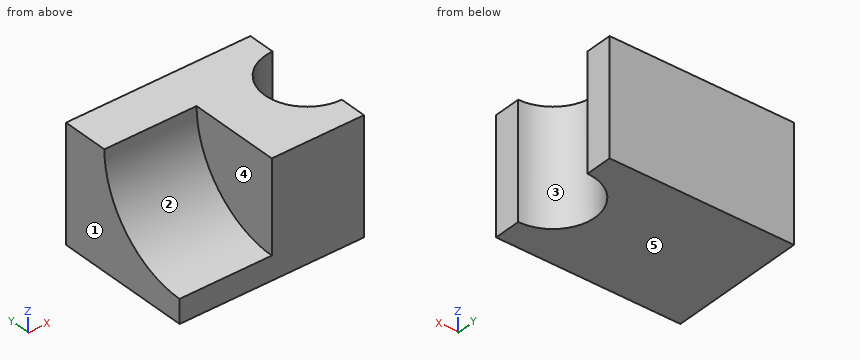
from build123d import *

# Parameters (mm, degrees)
F0_W     = 101.6
F0_H     = 76.2
F1_DEPTH = 63.5
F3_DEPTH = 71.628
F4_R     = 50.467154
F5_DEPTH = 50.8


with BuildPart() as f1:
    # F0 (on Top) → F1 (new body)
    with BuildSketch(Plane.XY):
        with Locations((83.7779, -52.045282)):
            Rectangle(F0_W, F0_H)
    extrude(amount=F1_DEPTH)

    # F2 (on face) → F3 (cut)
    with BuildSketch(Plane.XY.offset(63.5)):
        with BuildLine():
            ThreePointArc((134.5779, -75.284243), (151.010327, -68.477709), (157.81686, -52.045282))
            ThreePointArc((157.81686, -52.045282), (151.010327, -35.612856), (134.5779, -28.806322))
            Line((134.5779, -28.806322), (134.5779, -75.284243))
        make_face()
        with BuildLine():
            Line((134.5779, -75.284243), (134.5779, -28.806322))
            ThreePointArc((134.5779, -28.806322), (111.33894, -52.045282), (134.5779, -75.284243))
        make_face()
    extrude(amount=-F3_DEPTH, mode=Mode.SUBTRACT)

    # F4 (on face) → F5 (cut)
    with BuildSketch(Plane(origin=(32.9779, 0, 0), x_dir=(0, -1, 0), z_dir=(-1, 0, 0))):
        with Locations((90.145282, 63.5)):
            Circle(F4_R)
    extrude(amount=-F5_DEPTH, mode=Mode.SUBTRACT)


solid = f1.part
Design review of the part built by this model. Coordinates are the model's own, in mm. Face numbers are marked on the shaded views. A direction names the side the tool comes from. Coordinates: 2 decimals unless noted, no trailing zeros. Loops run counter-clockwise (first coordinate to the right, second up) from the corner with the lowest first, then second, coordinate; pieces in that order, holes last. Notation, with made-up numbers: M 36.25,-2 L 44.25,-2 A24 ccw 44.25,35 Z; hole C 79.5,-8.75 d3. An arc over 180 degrees is marked long. Use one line per item in the form item = value.
(1) Clearance check with flat-ended pins moving along their axes: P1, Ø15, axis at y = -66, z = 48.5, coming from the -X side; P2, Ø1.5, axis at y = -72.5, z = 26, coming from the +X side. State where each tip first meets the part, or that it passes through.
Return value:
P1 = 83.78
P2 = 125.07
(2) Draft analysis for pull direction Y (two halves, no side actions). For the marked faces 1, 2 and 3, state which applies: pulls with the +Y half, pulls with the -Y half, needs draft (parallel to the pull), parting line crosses it, or undercut.
Return value:
face_1 = needs draft
face_2 = pulls with the -Y half
face_3 = undercut
(3) Consider section D-D (y = -74). Write out the cut boundary in (x, z).
Return value:
outline = M 32.98,0 L 126.96,0 L 126.96,63.5 L 83.78,63.5 L 83.78,15.69 L 32.98,15.69 Z
(4) For the marked faces 4 and 5, list the 3-axis set-ups (+Z, -Z, +X, -X, +Y, -Y) from which the entire face can be reached by the end or side of a thin tool; tool diameter is ignored.
Return value:
face_4 = +Z, -X, -Y
face_5 = -Z, +X, -X, +Y, -Y
(5) For line 1 along X through (y, z) = (-86, 19.5); line 2 along Y through (x, z) = (130.5, 45); line 3 along Y through (x, z) = (116, 11.5), list the stretches that pass through material, from the lowest coordinate up. Write a range as from..to.
Return value:
line_1 = 83.78..134.58
line_2 = -90.15..-74.92, -29.17..-13.95
line_3 = -90.15..-66.01, -38.08..-13.95
(6) Consider section A-A (x = 43.5). Write out the cut boundary in (y, z).
Return value:
outline = M -90.15,0 L -13.95,0 L -13.95,63.5 L -39.68,63.5 A50.47 cw -90.15,13.03 Z
(7) Consider section C-C (x = 124). Write out the cut boundary in (y, z), and give its area (3 significant figures).
Return value:
outline = M -90.15,0 L -72.74,0 L -72.74,63.5 L -90.15,63.5 Z; M -31.35,0 L -13.95,0 L -13.95,63.5 L -31.35,63.5 Z
area = 2,210 mm2
